```python
from build123d import *

# Parameters (mm, degrees)
BOSS_EXTRUDE1_DEPTH = 3
BOSS_EXTRUDE2_DEPTH = 3
SKETCH3_R           = 2.9
CUT_EXTRUDE1_DEPTH  = 2
SKETCH4_R           = 1.5
CUT_EXTRUDE2_DEPTH  = 31.164382971
SKETCH8_R           = 1.5
CUT_EXTRUDE4_DEPTH  = 31.901294471


# Read off the part's stored shape, not the designer's step: Boss-Extrude2
with BuildPart() as part:
    # Sketch1 → Boss-Extrude1 (new body)
    with BuildSketch(Plane(origin=(0, 0, 0), x_dir=(1, 0, 0), z_dir=(0, 1, 0))):
        with BuildLine():
            Line((10.062305899, 3), (20.354248689, 3))
            ThreePointArc((20.354248689, 3), (27, 0), (20.354248689, -3))
            Line((20.354248689, -3), (10.062305899, -3))
            ThreePointArc((10.062305899, -3), (-10.5, 0), (10.062305899, 3))
        make_face()
    extrude(amount=BOSS_EXTRUDE1_DEPTH)

    # Boss-Extrude2 outline → Boss-Extrude2 (add)
    with BuildSketch(Plane(origin=(0, 0, 0), x_dir=(1, 0, 0), z_dir=(0, 1, 0))):
        with BuildLine():
            ThreePointArc((-10.969752428, 0.043811644), (-10.62658841, -0.230674076), (-10.480170576, -0.64499976))
            ThreePointArc((-10.480170576, -0.64499976), (-10.419978693, 1.293848534), (-10.00416019, 3.188538678))
            ThreePointArc((-10.00416019, 3.188538678), (-10.247462878, 2.822604668), (-10.647336332, 2.640381949))
            Line((-10.647336332, 2.640381949), (-12.457605143, 2.367968327))
            ThreePointArc((-12.457605143, 2.367968327), (-13.325815839, 1.778572113), (-12.863493028, 0.836534254))
            Line((-12.863493028, 0.836534254), (-12.861422527, 0.835664125))
            Line((-12.861422527, 0.835664125), (-10.969752428, 0.043811644))
        make_face()
        with BuildLine():
            ThreePointArc((-10.243204649, -3.926085368), (-9.824003519, -4.057898639), (-9.53766434, -4.391236606))
            ThreePointArc((-9.53766434, -4.391236606), (-10.18268144, -2.561835023), (-10.480170576, -0.64499976))
            ThreePointArc((-10.480170576, -0.64499976), (-10.574676775, -1.074152903), (-10.881592069, -1.388647488))
            Line((-10.881592069, -1.388647488), (-12.470837309, -2.297262873))
            ThreePointArc((-12.470837309, -2.297262873), (-13.067150653, -3.16073731), (-12.295452057, -3.87183434))
            Line((-12.295452057, -3.87183434), (-12.293207019, -3.871896838))
            Line((-12.293207019, -3.871896838), (-10.243204649, -3.926085368))
        make_face()
        with BuildLine():
            ThreePointArc((-8.130214562, -7.364577311), (-7.691719937, -7.33587578), (-7.304217543, -7.543103214))
            ThreePointArc((-7.304217543, -7.543103214), (-8.567135584, -6.070765016), (-9.53766434, -4.391236606))
            ThreePointArc((-9.53766434, -4.391236606), (-9.470582821, -4.825521696), (-9.64299823, -5.229720158))
            Line((-9.64299823, -5.229720158), (-10.796111745, -6.651554034))
            ThreePointArc((-10.796111745, -6.651554034), (-11.039815297, -7.672233361), (-10.06319217, -8.056140874))
            Line((-10.06319217, -8.056140874), (-10.061076468, -8.055387281))
            Line((-10.061076468, -8.055387281), (-8.130214562, -7.364577311))
        make_face()
        with BuildLine():
            ThreePointArc((-4.916780441, -9.806256059), (-4.518336336, -9.620925825), (-4.08211637, -9.674002581))
            ThreePointArc((-4.08211637, -9.674002581), (-5.792005958, -8.758005879), (-7.304217543, -7.543103214))
            ThreePointArc((-7.304217543, -7.543103214), (-7.084623431, -7.923740715), (-7.099201461, -8.362937666))
            Line((-7.099201461, -8.362937666), (-7.660106573, -10.105541409))
            ThreePointArc((-7.660106573, -10.105541409), (-7.518214471, -11.145274231), (-6.468855097, -11.150029425))
            Line((-6.468855097, -11.150029425), (-6.467155094, -11.148561743))
            Line((-6.467155094, -11.148561743), (-4.916780441, -9.806256059))
        make_face()
        with BuildLine():
            ThreePointArc((-1.037848299, -10.920634538), (-0.733386184, -10.603757733), (-0.307489921, -10.495496651))
            ThreePointArc((-0.307489921, -10.495496651), (-2.232907068, -10.259830702), (-4.08211637, -9.674002581))
            ThreePointArc((-4.08211637, -9.674002581), (-3.739741201, -9.949469528), (-3.594510754, -10.364211511))
            Line((-3.594510754, -10.364211511), (-3.48728761, -12.191719526))
            ThreePointArc((-3.48728761, -12.191719526), (-2.979005292, -13.109775513), (-1.998942976, -12.734734761))
            Line((-1.998942976, -12.734734761), (-1.997888773, -12.732751643))
            Line((-1.997888773, -12.732751643), (-1.037848299, -10.920634538))
        make_face()
        with BuildLine():
            ThreePointArc((2.981559098, -10.556878949), (3.150822189, -10.151350876), (3.508737967, -9.896401259))
            ThreePointArc((3.508737967, -9.896401259), (1.628412136, -10.372958783), (-0.307489921, -10.495496651))
            ThreePointArc((-0.307489921, -10.495496651), (0.111325954, -10.628511574), (0.396705602, -10.962664478))
            Line((0.396705602, -10.962664478), (1.157544092, -12.627719175))
            ThreePointArc((1.157544092, -12.627719175), (1.963419396, -13.299837247), (2.741530869, -12.595763214))
            Line((2.741530869, -12.595763214), (2.741796583, -12.59353308))
            Line((2.741796583, -12.59353308), (2.981559098, -10.556878949))
        make_face()
        with BuildLine():
            Line((7.031129829, -10.903441128), (6.281480785, -8.413857567))
            ThreePointArc((6.281480785, -8.413857567), (4.950917062, -9.25950432), (3.508737967, -9.896401259))
            ThreePointArc((3.508737967, -9.896401259), (3.947316897, -9.868954826), (4.334226904, -10.077294525))
            Line((4.334226904, -10.077294525), (5.804964161, -11.509633365))
            ThreePointArc((5.804964161, -11.509633365), (6.588651042, -11.551623858), (7.031129829, -10.903441128))
        make_face()
    extrude(amount=BOSS_EXTRUDE2_DEPTH)

    # Sketch3 → Cut-Extrude1 (cut)
    with BuildSketch(Plane(origin=(0, 3, 0), x_dir=(1, 0, 0), z_dir=(0, 1, 0))):
        with Locations(Location((23, 0, 0), (0, 0, 270))):
            Circle(SKETCH3_R)
    extrude(amount=-CUT_EXTRUDE1_DEPTH, mode=Mode.SUBTRACT)

    # Sketch4 → Cut-Extrude2 (cut, through all)
    with BuildSketch(Plane(origin=(0, 1, 0), x_dir=(1, 0, 0), z_dir=(0, 1, 0))):
        with Locations(Location((23, 0, 0), (0, 0, 270))):
            Circle(SKETCH4_R)
    extrude(amount=-CUT_EXTRUDE2_DEPTH, mode=Mode.SUBTRACT)

    # Sketch7 → Revolve1 (revolve)
    with BuildSketch(Plane.XY, mode=Mode.PRIVATE) as revolve1_sk:
        Polygon((2.75, 3), (9.5, 3), (6, 10), (2.75, 10), align=None)
    revolve(revolve1_sk.sketch.rotate(Axis((0, 0, 0), (0, 1, 0)), 90), axis=Axis((0, 0, 0), (0, 1, 0)))

    # Sketch8 → Cut-Extrude4 (cut, through all)
    with BuildSketch(Plane(origin=(0, 3, 0), x_dir=(1, 0, 0), z_dir=(0, 1, 0))):
        with Locations(Location((0, 0, 0), (0, 0, 270))):
            Circle(SKETCH8_R)
    extrude(amount=-CUT_EXTRUDE4_DEPTH, mode=Mode.SUBTRACT)


solid = part.part
```
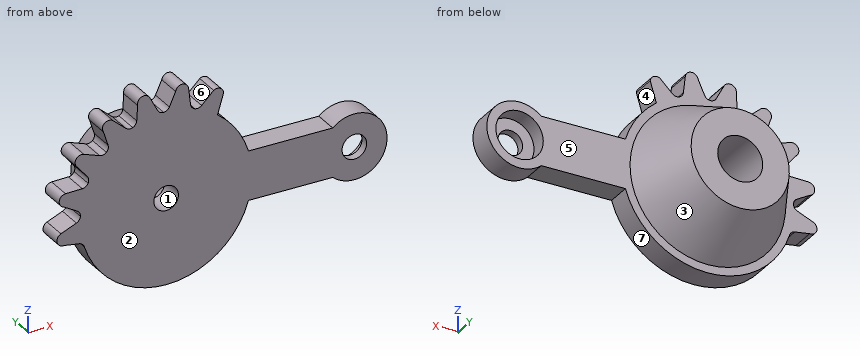
Verification items for the finished model (mm, model axes). Face numbers are marked on the shaded views. A direction names the side the tool comes from. Round coordinates to 2 decimals unless told otherwise and drop trailing zeros. Write each loop counter-clockwise with the first axis right and the second up, starting at its lowest first coordinate (ties: lowest second). Pieces come first, ordered by that corner, then holes. Notation, with made-up numbers: (43.5, 12) - (94.5, 12) arc R21 cw to (94.5, 32) - close; hole circle Ø1 at (-30.5, 14.25). An arc over 180 degrees is marked (long way). Answer as a JSON object with one key per item and string values. Group by question number.
Q1. Section check C-C, the plane y = 2.5. Give the number of separate pieces and of enclosed holes in the cut face, plus the area to 3 significant figures.
Q2. Section check D-D, the plane x = 17. Enter the section's corners in (y, z), plus the area to 3 significant figures.
Q3. Thickness scan on line 1 (X direction, y = 2.25, z = 0); line 2 (X direction, y = 0.5, z = 0); line 3 (X direction, y = 1.75, z = 2). Record the ranges inside material, lowest first.
Q4. Section check B-B, the plane y = 5. Enter the section's corners in (x, z), plus the area to 3 significant figures.
Q5. Go/stop test with flat-tipped pins: pin 1 Ø4 at (x, z) = (23, 0) entering from +Y; pin 2 Ø2 at (y, z) = (1.5, 4) entering from -X; pin 3 Ø3 at (x, y) = (2, 3.5) entering from -Z. Record where each tip stops, or that it passes through.
Q6. Tool access check on the marked faces 4, 5, 6 and 7. Record the directions out of +Z, -Z, +X, -X, +Y, -Y that give a thin tool (end or side, any length) a straight path to the whole face; none if there is none.
Q7. Section check A-A, the plane x = 23. Enter the section's corners in (y, z).
Q8. Mould release check, pull along X, two halves, no side actions. Record for the marked faces 1, 2 and 3: released by +X, released by -X, zero draft, split by the parting line, or undercut.
Found:
{
 "1": {"separate pieces": "1", "enclosed holes": "2", "area": "459 mm^2"},
 "2": {"outline": "(0, -3) - (3, -3) - (3, 3) - (0, 3) - close", "area": "18.0 mm^2"},
 "3": {"line 1": "x = -10.88 to -1.5, 1.5 to 20.1, 25.9 to 27", "line 2": "x = -10.88 to -1.5, 1.5 to 21.5, 24.5 to 27", "line 3": "x = -11.95 to 20.9, 25.1 to 26.46"},
 "4": {"outline": "circle Ø17 at (0, 0); hole circle Ø5.5 at (0, 0)", "area": "203 mm^2"},
 "5": {"pin 1": "stops at y = 1", "pin 2": "stops at x = -13.07", "pin 3": "stops at z = -10.48"},
 "6": {"face 4": "+X, +Y, -Y", "face 5": "+Y", "face 6": "+Z, +Y, -Y", "face 7": "-Z, +Y, -Y"},
 "7": {"outline": "(0, -4) - (3, -4) - (3, -2.9) - (1, -2.9) - (1, -1.5) - (0, -1.5) - close; (0, 1.5) - (1, 1.5) - (1, 2.9) - (3, 2.9) - (3, 4) - (0, 4) - close"},
 "8": {"face 1": "undercut", "face 2": "zero draft", "face 3": "split by the parting line"}
}
